Verification items for this drawing (mm, ordinates from the low corner). Give positions to 0.01 mm unless a question says otherwise; leave off trailing zeros. Order: outer loops, then holes, each group sorted by start corner. A loop starts at its lowest first (then second) coordinate and runs counter-clockwise, first axis right, second up. Notation, with made-up numbers: M 18,3 L 43,3 A21 ccw 43,14 Z; hole C 57.5,47 d1. An arc over 180 degrees is marked long. Answer as a JSON object with one key per item and string values.
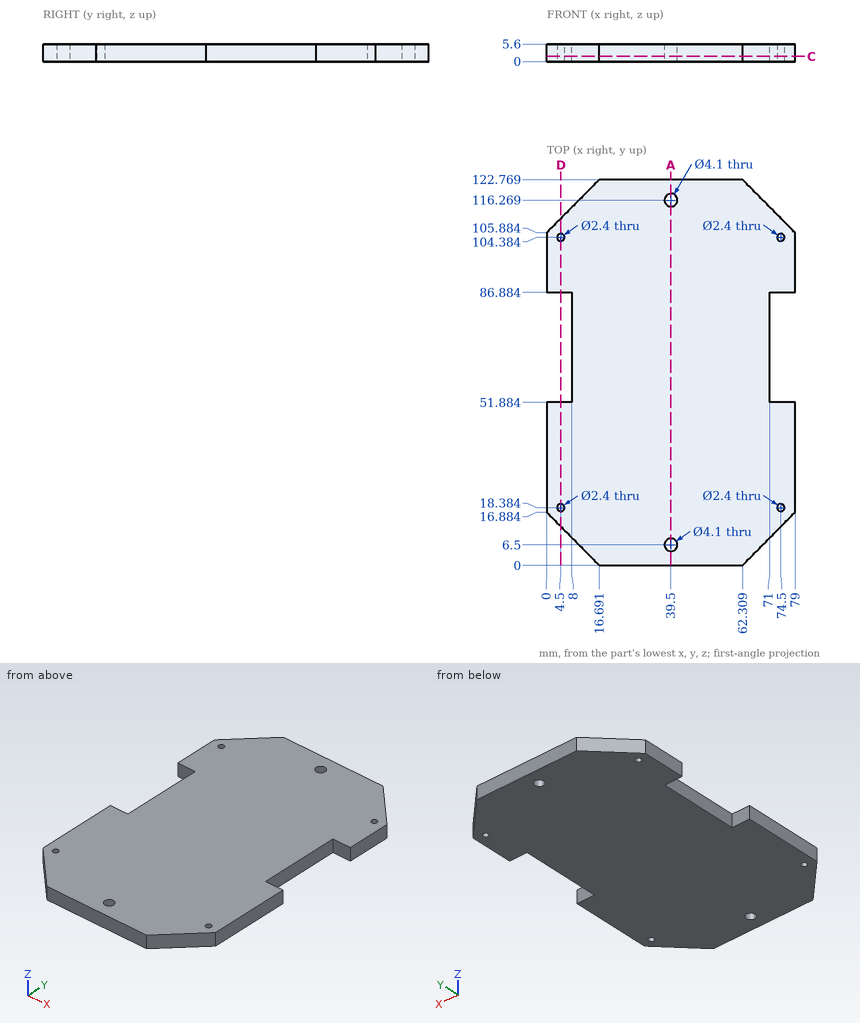
Q1. Section check D-D on x = 4.5. Record the cut outline in (y, z) (1 decimal).
Resolved:
{"outline": "M 12.3,0 L 17.2,0 L 17.2,5.6 L 12.3,5.6 Z; M 19.6,0 L 51.9,0 L 51.9,5.6 L 19.6,5.6 Z; M 86.9,0 L 103.2,0 L 103.2,5.6 L 86.9,5.6 Z; M 105.6,0 L 110.4,0 L 110.4,5.6 L 105.6,5.6 Z"}
Q2. Section check C-C on z = 1.7. Count the separate pieces of the cut face and the enclosed holes in it, then the cut area to 3 significant figures.
Resolved:
{"separate pieces": "1", "enclosed holes": "6", "area": "8,530 mm²"}
Q3. Gauge pin test, flat ends, axial feed: pin 1 Ø3 at (y, z) = (69.5, 3.5) entering from -X; pin 2 Ø2.5 at (x, y) = (39.5, 116.27) entering from -Z; pin 3 Ø1.7 at (y, z) = (77.5, 2.5) entering from +X; pin 4 Ø3 at (x, z) = (73.5, 2) entering from -Y (1 decimal). Record the tip position at first contact, or that the pin passes through.
Resolved:
{"pin 1": "stops at x = 8", "pin 2": "passes through", "pin 3": "stops at x = 71", "pin 4": "stops at y = 9.8"}
Q4. Material ranges on L1, parallel to Y at x = 39.5, z = 2.15; L2, parallel to X at y = 104.5, z = 4.55 (1 decimal); L3, parallel to X at y = 105, z = 1, recorded low to high.
Resolved:
{"L1": "y = 0 to 4.45, 8.55 to 114.22, 118.32 to 122.77", "L2": "x = 0 to 3.3, 5.7 to 73.3, 75.7 to 79", "L3": "x = 0 to 3.47, 5.53 to 73.47, 75.53 to 79"}
Q5. Section check A-A on x = 39.5. Record the cut outline in (y, z).
Resolved:
{"outline": "M 0,0 L 4.45,0 L 4.45,5.6 L 0,5.6 Z; M 8.55,0 L 114.22,0 L 114.22,5.6 L 8.55,5.6 Z; M 118.32,0 L 122.77,0 L 122.77,5.6 L 118.32,5.6 Z"}
